Source: CAD feature listing. Evaluate the final solid. Frame: model axes, mm. A direction names the side the tool comes from. Give positions to 0.01 mm unless a question says otherwise; leave off trailing zeros. Order: outer loops, then holes, each group sorted by start corner. A loop starts at its lowest first (then second) coordinate and runs counter-clockwise, first axis right, second up. Notation, with made-up numbers: M -18.5,48.25 L 12.5,48.25 A23 cw 12.5,63.25 Z; hole C 0.5,85.5 d1. An arc over 180 degrees is marked long. Return JSON: item names as keys, results as strings.
from build123d import *

# Parameters (mm, degrees)
SKETCH_1_W          = 12
SKETCH_1_H          = 12
EXTRUDE_1_DEPTH     = 9.5
SKETCH_2_R          = 5.5
EXTRUDE_2_DEPTH     = 54.5
SKETCH_3_W          = 12
SKETCH_3_H          = 12
EXTRUDE_3_DEPTH     = 12.5
SKETCH_4_R          = 4
EXTRUDE_4_DEPTH     = 8
SKETCH_5_R          = 2
CUT_EXTRUDE_1_DEPTH = 83.5
CUT_EXTRUDE_START   = -6
SKETCH_6_R          = 2.5
CUT_EXTRUDE_2_DEPTH = 6
FILLET_1_R          = 2


with BuildPart() as part:
    # 草图1 → 凸台-拉伸1 (new body)
    with BuildSketch(Plane.XY):
        Rectangle(SKETCH_1_W, SKETCH_1_H)
    extrude(amount=EXTRUDE_1_DEPTH)

    # 草图2 → 凸台-拉伸2 (add)
    with BuildSketch(Plane.XY.offset(9.5)):
        Circle(SKETCH_2_R)
    extrude(amount=EXTRUDE_2_DEPTH)

    # 草图3 → 凸台-拉伸3 (add)
    with BuildSketch(Plane.XY.offset(64)):
        Rectangle(SKETCH_3_W, SKETCH_3_H)
    extrude(amount=EXTRUDE_3_DEPTH)

    # 草图4 → 凸台-拉伸4 (add)
    with BuildSketch(Plane.XY.offset(76.5)):
        Circle(SKETCH_4_R)
    extrude(amount=EXTRUDE_4_DEPTH)

    # 草图5 → 切除-拉伸1 (cut)
    with BuildSketch(Plane.XY.offset(84.5)):
        Circle(SKETCH_5_R)
    extrude(amount=-CUT_EXTRUDE_1_DEPTH, mode=Mode.SUBTRACT)

    # 草图6 → 切除-拉伸2 (cut)
    with BuildSketch(Plane(origin=(0, 6, 0), x_dir=(1, 0, 0), z_dir=(0, 1, 0)).offset(CUT_EXTRUDE_START)):
        with Locations((0, -4.75)):
            Circle(SKETCH_6_R)
        with Locations((0, -68.75)):
            Circle(SKETCH_6_R)
    extrude(amount=CUT_EXTRUDE_2_DEPTH, mode=Mode.SUBTRACT)

    # 圆角1
    fillet_1_edges = [part.edges().sort_by_distance(p)[0] for p in [
        (6, -6, 70.25),
        (6, 6, 70.25),
        (-6, 6, 70.25),
        (-6, -6, 70.25),
        (6, -6, 4.75),
        (-6, -6, 4.75),
        (-6, 6, 4.75),
        (6, 6, 4.75),
    ]]
    fillet(fillet_1_edges, radius=FILLET_1_R)


solid = part.part
1. Section query C-C (y = -1). Return loops of the section in (x, z).
Evaluation:
{"outline": "M -6,0 L 6,0 L 6,9.5 L 5.41,9.5 L 5.41,64 L 6,64 L 6,76.5 L 3.87,76.5 L 3.87,84.5 L 1.73,84.5 L 1.73,1 L -1.73,1 L -1.73,84.5 L -3.87,84.5 L -3.87,76.5 L -6,76.5 L -6,64 L -5.41,64 L -5.41,9.5 L -6,9.5 Z"}
2. Set-up query: faces 4 (the face through (-3, -5, 9.5)), 5 (the face through (-6, 0, 70)), 6 (the face through (0, -2, 43)). Return all of +Z, -Z, +X, -X, +Y, -Y with unobstructed straight access to the full face (end or side cutting, diameter ignored); none if empty.
Evaluation:
{"face 4": "none", "face 5": "+Z, -Z, -X, +Y, -Y", "face 6": "+Z"}
3. Section query A-A (z = 75). Return loops of the section in (x, y).
Evaluation:
{"outline": "M -6,-4 A2 ccw -4,-6 L 4,-6 A2 ccw 6,-4 L 6,4 A2 ccw 4,6 L -4,6 A2 ccw -6,4 Z; hole C 0,0 d4"}
4. Section query D-D (z = 4.75). Return loops of the section in (x, y), then the cut area to 3 significant figures.
Evaluation:
{"outline": "M -6,-4 A2 ccw -4,-6 L 4,-6 A2 ccw 6,-4 L 6,4 A2 ccw 4,6 L 2.5,6 L 2.5,0 L 2,0 A2 cw -2,0 L -2.5,0 L -2.5,6 L -4,6 A2 ccw -6,4 Z", "area": "104 mm^2"}
5. Section query B-B (x = 0). Return loops of the section in (y, z), then the cut area to 4 significant figures.
Evaluation:
{"outline": "M -6,0 L 6,0 L 6,2.25 L 2,2.25 L 2,1 L -2,1 L -2,84.5 L -4,84.5 L -4,76.5 L -6,76.5 L -6,64 L -5.5,64 L -5.5,9.5 L -6,9.5 Z; M 2,7.25 L 6,7.25 L 6,9.5 L 5.5,9.5 L 5.5,64 L 6,64 L 6,66.25 L 2,66.25 Z; M 2,71.25 L 6,71.25 L 6,76.5 L 4,76.5 L 4,84.5 L 2,84.5 Z", "area": "553.5 mm^2"}
6. Draft query along Z for faces 1 (the face through (-2, -1, 84.5)), 2 (the face through (-2.498, 3.625, 4.64)), 3 (the face through (-0.867, -3.905, 80.444)). Return one class per face: pulls with the +Z half, pulls with the -Z half, needs draft (parallel to the pull), parting line crosses it, or undercut.
Evaluation:
{"face 1": "pulls with the +Z half", "face 2": "undercut", "face 3": "needs draft"}
7. First-contact query: pin 1 (0.6 mm diameter, centred on x = 2, z = 4.5, fed in from +Y); pin 2 (1.2 mm diameter, centred on x = 0, y = 1, fed in from +Z); pin 3 (2 mm diameter, centred on y = -4, z = 40.5, fed in from -X). Flat tips, straight axial feed; report the tip coordinate or a pass-through.
Evaluation:
{"pin 1": "stops at y = 0", "pin 2": "stops at z = 1", "pin 3": "stops at x = -4.61"}
8. Ray query, probe 1 along Z at (x, y) = (0, 3); probe 2 along Z at (x, y) = (0, 4.5); probe 3 along Z at (x, y) = (4, -5.25). Return the intervals inside material, ascending.
Evaluation:
{"probe 1": "z = 0 to 2.25, 7.25 to 66.25, 71.25 to 84.5", "probe 2": "z = 0 to 2.25, 7.25 to 66.25, 71.25 to 76.5", "probe 3": "z = 0 to 9.5, 64 to 76.5"}
